Geometry check sheet. Reference: the model listing, model coordinates, mm. A direction names the side the tool comes from. Round coordinates to 2 decimals unless told otherwise and drop trailing zeros. Write each loop counter-clockwise with the first axis right and the second up, starting at its lowest first coordinate (ties: lowest second). Pieces come first, ordered by that corner, then holes. Notation, with made-up numbers: M 57.25,-13 L 108.25,-13 A32 ccw 108.25,19 Z; hole C 32,78 d11. An arc over 180 degrees is marked long. Use a Markdown table: item, result.
```python
from build123d import *

# Parameters (mm, degrees)
BOX034_W     = 284
BOX034_H     = 13
BOX034_DEPTH = 13
BOX011_W     = 13
BOX011_H     = 600
BOX011_DEPTH = 13
BOX007_W     = 600
BOX007_H     = 13
BOX007_DEPTH = 13
BOX010_W     = 13
BOX010_H     = 600
BOX010_DEPTH = 13


with BuildPart() as cube031:
    # Box034 → Box034 (new body)
    with BuildSketch(Plane(origin=(-137, 525, -20), x_dir=(1, 0, 0), z_dir=(0, 0, 1))):
        with Locations((142, 6.5)):
            Rectangle(BOX034_W, BOX034_H)
    extrude(amount=BOX034_DEPTH)


with BuildPart() as cube008:
    # Box011 → Box011 (new body)
    with BuildSketch(Plane(origin=(-150, -62, -20), x_dir=(1, 0, 0), z_dir=(0, 0, 1))):
        with Locations((6.5, 300)):
            Rectangle(BOX011_W, BOX011_H)
    extrude(amount=BOX011_DEPTH)


with BuildPart() as frame_front:
    # Box007 → Box007 (new body)
    with BuildSketch(Plane(origin=(-300, -75, -20), x_dir=(1, 0, 0), z_dir=(0, 0, 1))):
        with Locations((300, 6.5)):
            Rectangle(BOX007_W, BOX007_H)
    extrude(amount=BOX007_DEPTH)


with BuildPart() as frame_full:
    # Box010 → Box010 (new body)
    with BuildSketch(Plane(origin=(147, -62, -20), x_dir=(1, 0, 0), z_dir=(0, 0, 1))):
        with Locations((6.5, 300)):
            Rectangle(BOX010_W, BOX010_H)
    extrude(amount=BOX010_DEPTH)

    # Connect014: union Cube008, Frame_Front
    add(cube008.part)
    add(frame_front.part)

    # Connect015: union Cube031
    add(cube031.part)


solid = frame_full.part
```
Item 1: Go/stop test with flat-tipped pins: pin 1 (4 mm diameter, centred on x = -197.5, z = -15.5, fed in from +Y); pin 2 (4 mm diameter, centred on y = 355.5, z = -13, fed in from +X). Record where each tip stops, or that it passes through.
Outcome:
| item | result |
|---|---|
| pin 1 | stops at y = -62 |
| pin 2 | stops at x = 160 |
Item 2: Mould release check, pull along Y, two halves, no side actions. Record for faces 6 (the face through (-4, -75, -14)), 7 (the face through (3, -62, -14)), 8 (the face through (300, -69, -14)): +Y half, -Y half, draft (parallel to the pull), parting line (faces both ways), or undercut.
Outcome:
| item | result |
|---|---|
| face 6 | -Y half |
| face 7 | undercut |
| face 8 | draft |
Item 3: Access from +Z, -Z, +X, -X, +Y, -Y to the whole of each face (thin tool, end or side, straight path). Record for faces 1 (the face through (-300, -69, -14)), 2 (the face through (154, 165, -20)), 3 (the face through (160, 234, -14)), 4 (the face through (-137, 227, -14)), 5 (the face through (-226, -62, -14)).
Outcome:
| item | result |
|---|---|
| face 1 | +Z, -Z, -X, +Y, -Y |
| face 2 | -Z, +X, -X, +Y, -Y |
| face 3 | +Z, -Z, +X, +Y |
| face 4 | +Z, -Z |
| face 5 | +Z, -Z, -X, +Y |
Item 4: Cross-section at C-C, the plane z = -15. Record the cut outline in (x, y), and give its area (3 significant figures).
Outcome:
| item | result |
|---|---|
| outline | M -300,-75 L 300,-75 L 300,-62 L 160,-62 L 160,538 L -150,538 L -150,-62 L -300,-62 Z; hole M -137,-62 L 147,-62 L 147,525 L -137,525 Z |
| area | 27,100 mm2 |
Item 5: Cross-section at B-B, the plane y = 300. Record the cut outline in (x, z), and give its area (3 significant figures).
Outcome:
| item | result |
|---|---|
| outline | M -150,-20 L -137,-20 L -137,-7 L -150,-7 Z; M 147,-20 L 160,-20 L 160,-7 L 147,-7 Z |
| area | 338 mm2 |
Item 6: Cross-section at A-A, the plane x = 43.5. Record the cut outline in (y, z).
Outcome:
| item | result |
|---|---|
| outline | M -75,-20 L -62,-20 L -62,-7 L -75,-7 Z; M 525,-20 L 538,-20 L 538,-7 L 525,-7 Z |
Item 7: Material ranges on line 1 along X through (y, z) = (390, -16); line 2 along Y through (x, z) = (-87, -12); line 3 along Y through (x, z) = (184.5, -12.5), recorded low to high. Write a range as from..to.
Outcome:
| item | result |
|---|---|
| line 1 | x = -150..-137, 147..160 |
| line 2 | y = -75..-62, 525..538 |
| line 3 | y = -75..-62 |
Item 8: Cross-section at D-D, the plane x = 238. Record the cut outline in (y, z).
Outcome:
| item | result |
|---|---|
| outline | M -75,-20 L -62,-20 L -62,-7 L -75,-7 Z |
